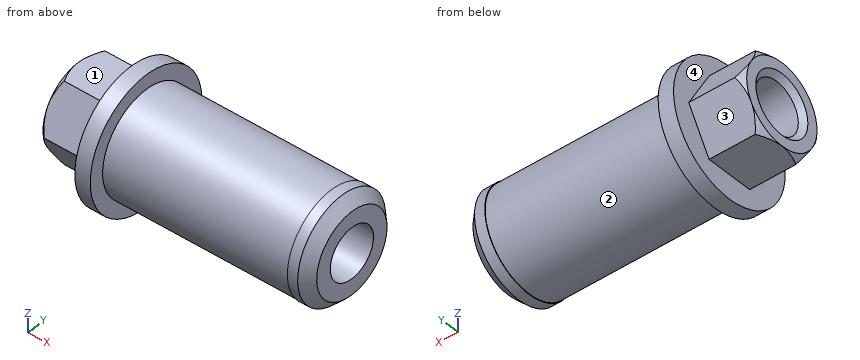
from build123d import *

# Parameters (mm, degrees)
SFAZOWANIE1_SIZE            = 1
SZKIC2_R                    = 2.46
DODANIE_WYCI_GNI_CIE1_DEPTH = 5.1
SFAZOWANIE2_SIZE            = 0.5


with BuildPart() as part:
    # Szkic1 → Obrót1 (revolve)
    with BuildSketch(Plane(origin=(0, 0, 0), x_dir=(1, 0, 0), z_dir=(0, 1, 0))):
        Polygon((0, 2.46), (0, 6.35), (1.5, 6.35), (1.5, 4.95), (19.5, 4.95), (19.5, 5), (21.5, 5), (21.5, 2.46), align=None)
    revolve(axis=Axis((0, 0, 0), (1, 0, 0)))

    # Sfazowanie1
    sfazowanie1_edges = [part.edges().sort_by_distance(p)[0] for p in [
        (21.5, 0, 5),
    ]]
    chamfer(sfazowanie1_edges, length=SFAZOWANIE1_SIZE)

    # Szkic2 → Dodanie-wyciągnięcie1 (add)
    with BuildSketch(Plane.ZY):
        Polygon((4, -2.309401077), (4, 2.309401077), (0, 4.618802154), (-4, 2.309401077), (-4, -2.309401077), (0, -4.618802154), align=None)
        Circle(SZKIC2_R, mode=Mode.SUBTRACT)
    extrude(amount=DODANIE_WYCI_GNI_CIE1_DEPTH)

    # Szkic3 → Wycięcie-obrót1 (revolve, cut)
    with BuildSketch(Plane.XY):
        Polygon((-5.1, 4.618802154), (-4.481197846, 4.618802154), (-5.1, 4), align=None)
    revolve(axis=Axis((-4.836570642, 0, 0), (-1, 0, 0)), mode=Mode.SUBTRACT)

    # Sfazowanie2
    sfazowanie2_edges = [part.edges().sort_by_distance(p)[0] for p in [
        (-5.1, 0, -2.46),
    ]]
    chamfer(sfazowanie2_edges, length=SFAZOWANIE2_SIZE)


solid = part.part
Verification items for the finished model (mm, model axes). Face numbers are marked on the shaded views. A direction names the side the tool comes from. Coordinates: 2 decimals unless noted, no trailing zeros. Write each loop counter-clockwise with the first axis right and the second up, starting at its lowest first coordinate (ties: lowest second). Pieces come first, ordered by that corner, then holes. Notation, with made-up numbers: (43, 52) - (65, 52) arc R31 cw to (65, 78) - close; hole circle Ø9 at (60, 42.5). An arc over 180 degrees is marked (long way). Answer as a JSON object with one key per item and string values.
(1) Thickness scan on line 1 along Z through (x, y) = (-1.55, 0); line 2 along Y through (x, z) = (8.75, 0); line 3 along Y through (x, z) = (2.25, -1.5). Record the ranges inside material, lowest first.
Report:
{"line 1": "-4 to -2.46, 2.46 to 4", "line 2": "-4.95 to -2.46, 2.46 to 4.95", "line 3": "-4.72 to -1.95, 1.95 to 4.72"}
(2) Cross-section at B-B on x = 9.75. Record the cut outline in (y, z).
Report:
{"outline": "circle Ø9.9 at (0, 0); hole circle Ø4.92 at (0, 0)"}
(3) Cross-section at A-A on x = 0.5. Record the cut outline in (y, z).
Report:
{"outline": "circle Ø12.7 at (0, 0); hole circle Ø4.92 at (0, 0)"}
(4) Gauge pin test, flat ends, axial feed: pin 1 Ø1 at (x, z) = (6, 5) entering from -Y; pin 2 Ø1.4 at (x, y) = (-2, -1) entering from -Z; pin 3 Ø2 at (x, y) = (3, 0) entering from +Z. Record the tip position at first contact, or that the pin passes through.
Report:
{"pin 1": "y = -2.06", "pin 2": "z = -4", "pin 3": "z = 4.95"}
(5) Tool access check on the marked faces 1, 2, 3 and 4. Record the directions out of +Z, -Z, +X, -X, +Y, -Y that give a thin tool (end or side, any length) a straight path to the whole face; none if there is none.
Report:
{"face 1": "+Z, -X, +Y, -Y", "face 2": "none", "face 3": "-Z, -X, +Y", "face 4": "-X"}
(6) Cross-section at C-C on y = 5.5. Record the cut outline in (x, z).
Report:
{"outline": "(0, -3.17) - (1.5, -3.17) - (1.5, 3.17) - (0, 3.17) - close"}
